from build123d import *

# Parameters (mm, degrees)
SKETCH3_W           = 236.719908988
SKETCH3_H           = 211.092865268
BOSS_EXTRUDE2_DEPTH = 2
SKETCH4_R           = 34.5
CUT_EXTRUDE2_DEPTH  = 2
SKETCH5_W           = 236.719908988
SKETCH5_H           = 211.092865268
CUT_EXTRUDE3_DEPTH  = 2
SKETCH6_R           = 1.7
CUT_EXTRUDE4_DEPTH  = 2


with BuildPart() as part:
    # Sketch3 → Boss-Extrude2 (new body)
    with BuildSketch(Plane(origin=(0, 0, 0), x_dir=(1, 0, 0), z_dir=(0, 1, 0))):
        Rectangle(SKETCH3_W, SKETCH3_H)
    extrude(amount=BOSS_EXTRUDE2_DEPTH)

    # Sketch4 → Cut-Extrude2 (cut)
    with BuildSketch(Plane(origin=(0, 2, 0), x_dir=(1, 0, 0), z_dir=(0, 1, 0))):
        Circle(SKETCH4_R)
    extrude(amount=-CUT_EXTRUDE2_DEPTH, mode=Mode.SUBTRACT)

    # Sketch5 → Cut-Extrude3 (cut)
    with BuildSketch(Plane(origin=(0, 2, 0), x_dir=(1, 0, 0), z_dir=(0, 1, 0))):
        Rectangle(SKETCH5_W, SKETCH5_H)
        with BuildLine():
            ThreePointArc((6.370089382, 37.28475005), (26.746313998, 26.746313998), (37.28475005, 6.370089382))
            ThreePointArc((37.28475005, 6.370089382), (44.217957746, 0), (37.28475005, -6.370089382))
            ThreePointArc((37.28475005, -6.370089382), (26.746313998, -26.746313998), (6.370089382, -37.28475005))
            ThreePointArc((6.370089382, -37.28475005), (0, -44.217957746), (-6.370089382, -37.28475005))
            ThreePointArc((-6.370089382, -37.28475005), (-26.746313998, -26.746313998), (-37.28475005, -6.370089382))
            ThreePointArc((-37.28475005, -6.370089382), (-44.217957746, 0), (-37.28475005, 6.370089382))
            ThreePointArc((-37.28475005, 6.370089382), (-26.746313998, 26.746313998), (-6.370089382, 37.28475005))
            ThreePointArc((-6.370089382, 37.28475005), (0, 44.217957746), (6.370089382, 37.28475005))
        make_face(mode=Mode.SUBTRACT)
    extrude(amount=-CUT_EXTRUDE3_DEPTH, mode=Mode.SUBTRACT)

    # Sketch6 → Cut-Extrude4 (cut)
    with BuildSketch(Plane(origin=(0, 2, 0), x_dir=(1, 0, 0), z_dir=(0, 1, 0))):
        with Locations((0, 40.133145431)):
            Circle(SKETCH6_R)
        with Locations((-40.133145431, 0)):
            Circle(SKETCH6_R)
        with Locations((0, -40.133145431)):
            Circle(SKETCH6_R)
        with Locations((40.133145431, 0)):
            Circle(SKETCH6_R)
    extrude(amount=-CUT_EXTRUDE4_DEPTH, mode=Mode.SUBTRACT)


solid = part.part
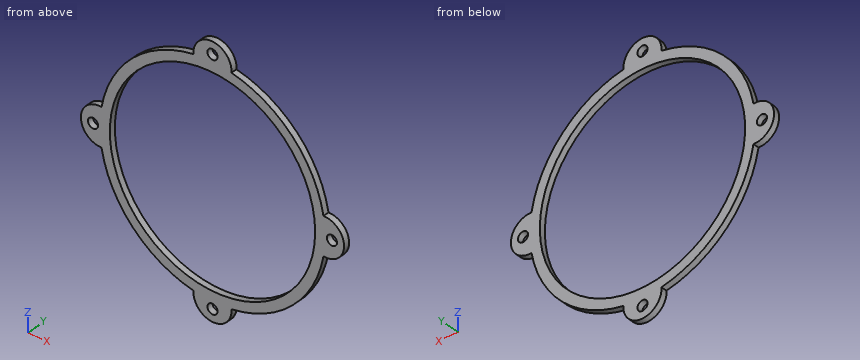
Geometry check sheet. Reference: the model listing, model coordinates, mm. Round coordinates to 2 decimals unless told otherwise and drop trailing zeros. Loops run counter-clockwise (first coordinate to the right, second up) from the corner with the lowest first, then second, coordinate; pieces in that order, holes last. Notation, with made-up numbers: (-13, 8) -> (-6, 8) arc R34 cw to (-6, 42) -> close; hole circle Ø7 at (86, -16.5). An arc over 180 degrees is marked (long way). Answer as a JSON object with one key per item and string values. Group by question number.
Item 1: Cross-section at B-B, the plane x = 0. Record the cut outline in (y, z).
Item 2: Thickness scan on line 1 along X through (y, z) = (0.8, 0); line 2 along X through (y, z) = (1.75, 21). Record the ranges inside material, lowest first.
Item 3: Cross-section at C-C, the plane z = -26.5. Record the cut outline in (x, y).
Item 4: Cross-section at D-D, the plane x = 23. Record the cut outline in (y, z), plus the area to 3 significant figures.
Item 5: Depth check by flat-ended pin: pin 1 Ø2.5 at (x, z) = (0, -40.13) entering from -Y. Enter the tip coordinate at first touch or a pass-through.
Item 6: Cross-section at A-A, the plane z = 0. Record the cut outline in (x, y), plus the area to 3 significant figures.
Determined:
{
 "1": {"outline": "(0, -44.22) -> (2, -44.22) -> (2, -41.83) -> (0, -41.83) -> close; (0, -38.43) -> (2, -38.43) -> (2, -34.5) -> (0, -34.5) -> close; (0, 34.5) -> (2, 34.5) -> (2, 38.43) -> (0, 38.43) -> close; (0, 41.83) -> (2, 41.83) -> (2, 44.22) -> (0, 44.22) -> close"},
 "2": {"line 1": "x = -44.22 to -41.83, -38.43 to -34.5, 34.5 to 38.43, 41.83 to 44.22", "line 2": "x = -31.46 to -27.37, 27.37 to 31.46"},
 "3": {"outline": "(-26.99, 0) -> (-22.09, 0) -> (-22.09, 2) -> (-26.99, 2) -> close; (22.09, 0) -> (26.99, 0) -> (26.99, 2) -> (22.09, 2) -> close"},
 "4": {"outline": "(0, -30.03) -> (2, -30.03) -> (2, -25.71) -> (0, -25.71) -> close; (0, 25.71) -> (2, 25.71) -> (2, 30.03) -> (0, 30.03) -> close", "area": "17.3 mm²"},
 "5": {"pin 1": "passes through"},
 "6": {"outline": "(-44.22, 0) -> (-41.83, 0) -> (-41.83, 2) -> (-44.22, 2) -> close; (-38.43, 0) -> (-34.5, 0) -> (-34.5, 2) -> (-38.43, 2) -> close; (34.5, 0) -> (38.43, 0) -> (38.43, 2) -> (34.5, 2) -> close; (41.83, 0) -> (44.22, 0) -> (44.22, 2) -> (41.83, 2) -> close", "area": "25.3 mm²"}
}
